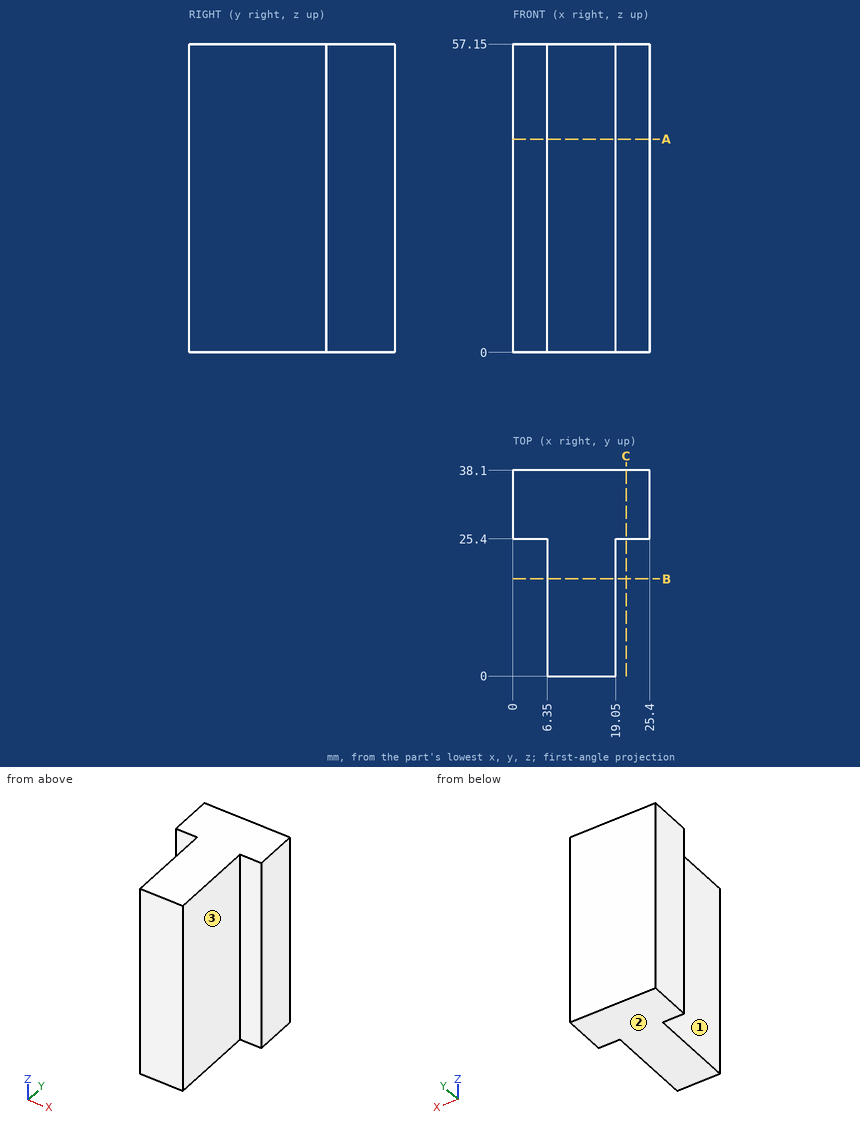
Drawing for the job (mm, zero at the part's lowest x, y, z). A direction names the side the tool comes from. Round coordinates to 2 decimals unless told otherwise and drop trailing zeros. Write each loop counter-clockwise with the first axis right and the second up, starting at its lowest first coordinate (ties: lowest second). Pieces come first, ordered by that corner, then holes. Notation, with made-up numbers: M 89,-13.5 L 120,-13.5 A14 cw 120,-6.5 Z; hole C -7,-34.5 d5. An arc over 180 degrees is marked long. Put each result on its own line as item: value.
Item 1: Cut at B-B (y = 18). List the corners of the cut face in (x, z), and give its area (3 significant figures).
Responses:
outline: M 6.35,0 L 19.05,0 L 19.05,57.15 L 6.35,57.15 Z
area: 726 mm²
Item 2: Cut at C-C (x = 21). List the corners of the cut face in (y, z), and give its area (3 significant figures).
Responses:
outline: M 25.4,0 L 38.1,0 L 38.1,57.15 L 25.4,57.15 Z
area: 726 mm²
Item 3: Probe L1, parallel to X at y = 15, z = 54; L2, parallel to Y at x = 24, z = 4. List the from-to ranges inside material, lowest first. Write a range as from..to.
Responses:
L1: 6.35..19.05
L2: 25.4..38.1
Item 4: Cut at A-A (z = 39.5). List the corners of the cut face in (x, y), and give its area (3 significant figures).
Responses:
outline: M 0,25.4 L 6.35,25.4 L 6.35,0 L 19.05,0 L 19.05,25.4 L 25.4,25.4 L 25.4,38.1 L 0,38.1 Z
area: 645 mm²
Item 5: Flat gauge pins, fed straight in: P1, Ø2, axis at x = 4.5, z = 14, coming from the -Y side; P2, Ø6, axis at y = 20.5, z = 31, coming from the +X side; P3, Ø12.5, axis at y = 11, z = 35, coming from the -X side; P4, Ø1.5, axis at x = 4, y = 6, coming from the +Z side (3 decimals). Where does each tip first touch, or does it go through?
Responses:
P1: y = 25.4
P2: x = 19.05
P3: x = 6.35
P4: through
Item 6: Tool access for the marked faces 1, 2 and 3: list every direction of +Z, -Z, +X, -X, +Y, -Y with a clear straight run to the whole face (end or side of a thin tool).
Responses:
face 1: +Z, -Z, -X, -Y
face 2: -Z, +X, -X, +Y, -Y
face 3: +Z, -Z, +X, -Y
